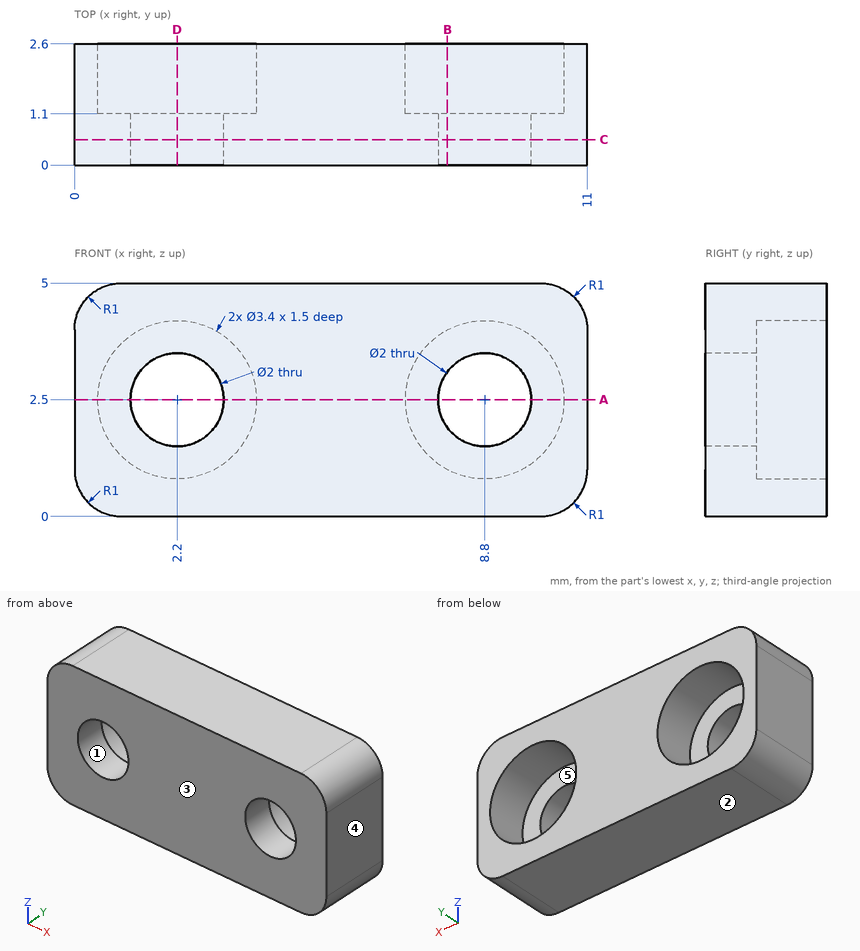
Geometry check sheet. Reference: drawing and pictorial views, mm from the part's lowest x, y, z. A direction names the side the tool comes from. Round coordinates to 2 decimals unless told otherwise and drop trailing zeros. Loops run counter-clockwise (first coordinate to the right, second up) from the corner with the lowest first, then second, coordinate; pieces in that order, holes last. Notation, with made-up numbers: M -13,-20 L 40,-20 A16 ccw 40,11 Z; hole C 69.25,84 d7. An arc over 180 degrees is marked long. Return JSON: item names as keys, results as strings. Group by question number.
(1) Section check C-C, the plane y = 0.55. Enter the section's corners in (x, z), and give its area (3 significant figures).
(2) Scan lines: line 1 along X through (y, z) = (1.85, 2.5); line 2 along X through (y, z) = (0.8, 2.5); line 3 along Z through (x, y) = (8.8, 1.65). Record each from-to range of solid material in increasing order. Write a range as [from, to].
(3) Section check D-D, the plane x = 2.2. Enter the section's corners in (y, z), and give its area (3 significant figures).
(4) Mould release check, pull along Z, two halves, no side actions. Record for the marked faces 1, 2 and 3: pulls with the +Z half, pulls with the -Z half, needs draft (parallel to the pull), parting line crosses it, or undercut.
(5) Section check A-A, the plane z = 2.5. Enter the section's corners in (x, y).
(6) Section check B-B, the plane x = 8. Enter the section's corners in (y, z).
(7) Go/stop test with flat-tipped pins: pin 1 (2 mm diameter, centred on x = 9, z = 3, fed in from -Y); pin 2 (1.7 mm diameter, centred on x = 9, z = 2.5, fed in from +Y); pin 3 (1.8 mm diameter, centred on x = 2.2, z = 2.5, fed in from -Y). Record where each tip stops, or that it passes through.
(8) Set-up check for the marked faces 4 and 5: record each of +Z, -Z, +X, -X, +Y, -Y from which the full face is reachable in a straight line by a thin tool's end or side.
Data:
{
 "1": {"outline": "M 0,1 A1 ccw 1,0 L 10,0 A1 ccw 11,1 L 11,4 A1 ccw 10,5 L 1,5 A1 ccw 0,4 Z; hole C 2.2,2.5 d2; hole C 8.8,2.5 d2", "area": "47.9 mm²"},
 "2": {"line 1": "[0, 0.5], [3.9, 7.1], [10.5, 11]", "line 2": "[0, 1.2], [3.2, 7.8], [9.8, 11]", "line 3": "[0, 0.8], [4.2, 5]"},
 "3": {"outline": "M 0,0 L 2.6,0 L 2.6,0.8 L 1.1,0.8 L 1.1,1.5 L 0,1.5 Z; M 0,3.5 L 1.1,3.5 L 1.1,4.2 L 2.6,4.2 L 2.6,5 L 0,5 Z", "area": "5.70 mm²"},
 "4": {"face 1": "undercut", "face 2": "pulls with the -Z half", "face 3": "needs draft"},
 "5": {"outline": "M 0,0 L 1.2,0 L 1.2,1.1 L 0.5,1.1 L 0.5,2.6 L 0,2.6 Z; M 3.2,0 L 7.8,0 L 7.8,1.1 L 7.1,1.1 L 7.1,2.6 L 3.9,2.6 L 3.9,1.1 L 3.2,1.1 Z; M 9.8,0 L 11,0 L 11,2.6 L 10.5,2.6 L 10.5,1.1 L 9.8,1.1 Z"},
 "6": {"outline": "M 0,0 L 2.6,0 L 2.6,1 L 1.1,1 L 1.1,1.9 L 0,1.9 Z; M 0,3.1 L 1.1,3.1 L 1.1,4 L 2.6,4 L 2.6,5 L 0,5 Z"},
 "7": {"pin 1": "y = 0", "pin 2": "y = 1.1", "pin 3": "through"},
 "8": {"face 4": "+Z, -Z, +X, +Y, -Y", "face 5": "+Y"}
}
